from build123d import *

# Parameters (mm, degrees)
F0_W     = 70
F0_H     = 40
F1_DEPTH = 63
F2_R     = 23.451483
F3_DEPTH = 74
F4_R     = 13.707811
F5_DEPTH = 87.035492
F6_R     = 15


with BuildPart() as f1:
    # F0 (on Top) → F1 (new body)
    with BuildSketch(Plane.XY):
        with Locations((0, -26)):
            Rectangle(F0_W, F0_H)
    extrude(amount=F1_DEPTH)

    # F2 (on face) → F3 (cut)
    with BuildSketch(Plane.XZ.offset(46)):
        with Locations((35, 63)):
            Circle(F2_R)
    extrude(amount=-F3_DEPTH, mode=Mode.SUBTRACT)

    # F4 (on Front) → F5 (cut)
    with BuildSketch(Plane.XZ):
        with Locations((-18.644467, 22.406071)):
            Circle(F4_R)
    extrude(amount=F5_DEPTH, mode=Mode.SUBTRACT)

    # F6
    f6_edges = [f1.edges().sort_by_distance(p)[0] for p in [
        (-11.725742, -46, 63),
    ]]
    fillet(f6_edges, radius=F6_R)


solid = f1.part
Input: part model. Units: mm. Frame: model coordinates. Coordinates: 2 decimals unless noted, no trailing zeros. Loops run counter-clockwise (first coordinate to the right, second up) from the corner with the lowest first, then second, coordinate; pieces in that order, holes last. Notation, with made-up numbers: (-32, 16) -> (9, 16) arc R11 cw to (9, 22) -> close; hole circle Ø1 at (66.5, 79). An arc over 180 degrees is marked (long way). One line per item, written item: value.
(1) Cut plane C-C (z = 33). Output: boundary loops of the cut face in (x, y).
Answer below:
outline: (-35, -46) -> (-27.34, -46) -> (-27.34, -6) -> (-35, -6) -> close; (-9.95, -46) -> (35, -46) -> (35, -6) -> (-9.95, -6) -> close
(2) Cut plane A-A (x = -30). Output: boundary loops of the cut face in (y, z), then the cut area to 3 significant figures.
Answer below:
outline: (-46, 0) -> (-6, 0) -> (-6, 14.73) -> (-46, 14.73) -> close; (-46, 30.08) -> (-6, 30.08) -> (-6, 63) -> (-31, 63) arc R15 ccw to (-46, 48) -> close
area: 1,860 mm2
(3) Cut plane D-D (y = -11). Output: boundary loops of the cut face in (x, z).
Answer below:
outline: (-35, 0) -> (35, 0) -> (35, 39.55) arc R23.45 cw to (11.55, 63) -> (-35, 63) -> close; hole circle Ø27.42 at (-18.64, 22.41)
(4) Ray query, line 1 along Z through (x, y) = (-11, -40); line 2 along X through (y, z) = (-26.5, 14.5); line 3 along X through (y, z) = (-14, 48). Return the intervals inside material, ascending.
Answer below:
line 1: z = 0 to 11.03, 33.78 to 60
line 2: x = -35 to -29.84, -7.45 to 35
line 3: x = -35 to 16.97
(5) Draft query along Z for faces 1 (the face through (0, -46, 24)), 2 (the face through (-28.75, -25.72, 31.67)), 3 (the face through (-12, -18, 63)), 4 (the face through (0, -26, 0)). Return one class per face: pulls with the +Z half, pulls with the -Z half, needs draft (parallel to the pull), parting line crosses it, or undercut.
Answer below:
face 1: needs draft
face 2: undercut
face 3: pulls with the +Z half
face 4: pulls with the -Z half
(6) Cut plane B-B (x = 1.5). Output: boundary loops of the cut face in (y, z), then the cut area to 3 significant figures.
Answer below:
outline: (-46, 0) -> (-6, 0) -> (-6, 63) -> (-31, 63) arc R15 ccw to (-46, 48) -> close
area: 2,470 mm2
